The model under review builds one solid part; all positions refer to its coordinate system, in mm. A direction names the side the tool comes from. Round coordinates to 2 decimals unless told otherwise and drop trailing zeros. Write each loop counter-clockwise with the first axis right and the second up, starting at its lowest first coordinate (ties: lowest second). Pieces come first, ordered by that corner, then holes. Notation, with made-up numbers: (71.5, 34.25) -> (78.5, 34.25) arc R17 cw to (78.5, 52.25) -> close; hole circle Ø1 at (-5, -27.75). An arc over 180 degrees is marked (long way). Use CSV: the item, a comma, the result in double quotes. Start each with the question number.
1) For pin 1 Ø0.6 at (y, z) = (-1, 24.5) entering from +X; pin 2 Ø0.6 at (x, z) = (1, 24.5) entering from +Y; pin 3 Ø0.6 at (x, z) = (-1, 24.5) entering from -Y, all flat-tipped, find the tip position at first contact; note any pin that passes through.
2) Machinability: for faces 1 (the face through (0, 0, 0)), 2 (the face through (0, -2, 24.1)), which of the approach directions +Z, -Z, +X, -X, +Y, -Y give a long, thin tool a straight path to every point of the face, cutting with its end or side? Answer none if there is none.
3) Take a section at A-A, the plane z = 3.75. Give the boundary of the cut face in (x, y).
4) Wall thickness on probe 1 along Z at (x, y) = (-1.35, -0.3); probe 2 along Y at (x, z) = (0.4, 23); probe 3 along Y at (x, z) = (0.3, 19.75): over which ranges is each line inside the solid? List them lowest first. Write a range as [from, to].
from build123d import *

# Parameters (mm, degrees)
F0_R     = 1.5
F1_DEPTH = 24.6
F2_R     = 2.61
F2_R_2   = 1.5
F3_DEPTH = 0.5
F5_DEPTH = 0.5


# Not quite as in the source:
# - a fillet or chamfer that OpenCascade refuses, or shapes differently, is made with other operations: its cross-section is extruded or revolved along the edge and cut away or added


with BuildPart() as f1:
    # F0 (on Top) → F1 (new body)
    with BuildSketch(Plane.XY):
        Circle(F0_R)
    extrude(amount=F1_DEPTH)

    # F2 (on face) → F3 (join)
    with BuildSketch(Plane.XY.offset(24.6)):
        Circle(F2_R)
        Circle(F2_R_2, mode=Mode.SUBTRACT)
    extrude(amount=-F3_DEPTH)

    # F4: fillet of radius 2 on 1 edges, made by hand

    # F4_s1 → F4_t2 (revolve, cut)
    with BuildSketch(Plane.XZ):
        with BuildLine():
            ThreePointArc((2.61, 24.1), (1.9942311257, 24.4708286934), (1.2871243445, 24.6))
            Line((1.2871243445, 24.6), (2.61, 24.6))
            Line((2.61, 24.6), (2.61, 24.1))
        make_face()
    revolve(axis=Axis((0, 0, 24.6), (0, 0, 1)), mode=Mode.SUBTRACT)

    # F2 (on face) → F5 (cut)
    with BuildSketch(Plane.XY.offset(24.6)):
        Polygon((-1.2485300168, 0.125), (-1.2485300168, -0.125), (-0.125, -0.125), (-0.125, -1.2485300168), (0.125, -1.2485300168), (0.125, -0.125), (1.2485300168, -0.125), (1.2485300168, 0.125), (0.125, 0.125), (0.125, 1.2485300168), (-0.125, 1.2485300168), (-0.125, 0.125), align=None)
    extrude(amount=-F5_DEPTH, mode=Mode.SUBTRACT)


solid = f1.part
Values found:
1,pin 1,"x = 2.29"
1,pin 2,"y = 2.29"
1,pin 3,"y = -2.29"
2,face 1,"-Z, +X, -X, +Y, -Y"
2,face 2,"-Z"
3,outline,"circle Ø3 at (0, 0)"
4,probe 1,"[0, 24.6]"
4,probe 2,"[-1.45, 1.45]"
4,probe 3,"[-1.47, 1.47]"
